Geometry check sheet. Reference: the model listing, model coordinates, mm. A direction names the side the tool comes from. Give positions to 0.01 mm unless a question says otherwise; leave off trailing zeros. Write each loop counter-clockwise with the first axis right and the second up, starting at its lowest first coordinate (ties: lowest second). Pieces come first, ordered by that corner, then holes. Notation, with made-up numbers: M -11.5,-4.75 L 8.5,-4.75 A29 cw 8.5,25.25 Z; hole C -15,48.5 d4. An arc over 180 degrees is marked long. Write each question's results on one line, items separated by ' | '.
```python
from build123d import *

# Parameters (mm, degrees)
CROQUIS1_R              = 2
SALIENTE_EXTRUIR1_DEPTH = 5


with BuildPart() as part:
    # Croquis1 → Saliente-Extruir1 (new body)
    with BuildSketch(Plane.XY):
        Polygon((0, 20), (5, 20), (5, 30), (52, 30), (52, 25), (104, 25), (104, 30), (156, 30), (156, 25), (208, 25), (208, 30), (255, 30), (255, 20), (260, 20), (260, 10), (255, 10), (255, 0), (208, 0), (208, 5), (156, 5), (156, 0), (104, 0), (104, 5), (52, 5), (52, 0), (5, 0), (5, 10), (0, 10), align=None)
        with Locations((16, 16)):
            Circle(CROQUIS1_R, mode=Mode.SUBTRACT)
        with Locations(Location((244, 16, 0), (0, 0, 180))):
            Circle(CROQUIS1_R, mode=Mode.SUBTRACT)
    extrude(amount=SALIENTE_EXTRUIR1_DEPTH)


solid = part.part
```
Q1. Section check B-B (x = 189). Enter the section's corners in (y, z).
Answer key:
outline: M 5,0 L 25,0 L 25,5 L 5,5 Z
Q2. Section check A-A (z = 3.65). State how many separate pieces and enclosed holes the cut face has, then the cut area to 3 significant figures.
Answer key:
separate pieces: 1 | enclosed holes: 2 | area: 6,530 mm2
Q3. Release check for a two-part mould opening along Y. For faces 5 (the face through (16, 18, 2)), 6 (the face through (255, 5, 2)), 7 (the face through (231, 30, 2)) record: released by +Y, released by -Y, zero draft, split by the parting line, or undercut.
Answer key:
face 5: undercut | face 6: zero draft | face 7: released by +Y
Q4. Access from +Z, -Z, +X, -X, +Y, -Y to the whole of each face (thin tool, end or side, straight path). Record for faces 1 (the face through (156, 28, 2)), 2 (the face through (156, 3, 2)), 3 (the face through (5, 25, 2)), 4 (the face through (257, 20, 2)).
Answer key:
face 1: +Z, -Z, +Y | face 2: +Z, -Z, -Y | face 3: +Z, -Z, -X, +Y | face 4: +Z, -Z, +X, +Y
Q5. Depth check by flat-ended pin: P1, Ø1.5, axis at y = 2.5, z = 3.5, coming from the +X side; P2, Ø1, axis at x = 180.5, z = 2.5, coming from the -Y side; P3, Ø3.5, axis at x = 244, y = 16, coming from the -Z side; P4, Ø1.5, axis at y = 28, z = 3, coming from the -X side. Enter the tip coordinate at first touch or a pass-through.
Answer key:
P1: stops at x = 255 | P2: stops at y = 5 | P3: passes through | P4: stops at x = 5
Q6. Material ranges on probe 1 along X at (y, z) = (25.5, 3.95); probe 2 along Y at (x, z) = (244, 3.55); probe 3 along X at (y, z) = (17.5, 3.1), recorded low to high. Write a range as [from, to].
Answer key:
probe 1: x = [5, 52], [104, 156], [208, 255] | probe 2: y = [0, 14], [18, 30] | probe 3: x = [0, 14.68], [17.32, 242.68], [245.32, 260]
